Model file for the job. Use its own axes, mm. Face numbers are marked on the shaded views. A direction names the side the tool comes from. Coordinates: 2 decimals unless noted, no trailing zeros. Write each loop counter-clockwise with the first axis right and the second up, starting at its lowest first coordinate (ties: lowest second). Pieces come first, ordered by that corner, then holes.
Q1. Pin check, flat tips, straight feed: P1, Ø2.5, axis at x = -35, z = -1, coming from the -Y side; P2, Ø6, axis at x = 15.5, z = -18, coming from the -Y side; P3, Ø1, axis at x = -40.5, z = -86, coming from the -Y side; P4, Ø6, axis at x = -2.5, y = 5.5, coming from the -Z side. Stop position of each tip, or through.
Q2. Which spindle directions (+Z, -Z, +X, -X, +Y, -Y) get a long thin tool onto all of the face, cutting with end or side? Do the marked faces 5 and 6. Say none if no direction does.
Q3. Band-saw the part on C-C, the plane x = -27.5. Write the cut outline in (y, z).
Q4. Band-saw the part on D-D, the plane z = -81. Write the cut outline in (x, y).
Q5. Pull direction X, two halves, no side cores. Call the marked faces 1, 2, 3 and 4: released by +X, released by -X, zero draft, split by the parting line, or undercut.
Q6. Drill centre lines: probe 1 along X at (y, z) = (22.5, -30.5); probe 2 along Y at (x, z) = (4, -94); probe 3 along Z at (x, y) = (-5.5, 32). Where is each one in solid material? Low to high.
Q7. Band-saw the part on B-B, the plane y = 25. Write the cut outline in (x, z), plus the area to 3 significant figures.
Q8. Band-saw the part on A-A, the plane z = -7. Write the cut outline in (x, y), plus the area to 4 significant figures.
from build123d import *

# Parameters (mm, degrees)
SALIENTE_EXTRUIR1_DEPTH = 107
CROQUIS2_W              = 90
CROQUIS2_H              = 18
SALIENTE_EXTRUIR2_DEPTH = 3
CROQUIS4_W              = 90
CROQUIS4_H              = 30
SALIENTE_EXTRUIR3_DEPTH = 3
REDONDEO3_R             = 2
CROQUIS3_W              = 6
CROQUIS3_H              = 45
CORTAR_EXTRUIR1_DEPTH   = 123.776219196
REDONDEO1_R             = 5
SALIENTE_EXTRUIR4_DEPTH = 3.5
CORTAR_EXTRUIR3_START   = -3
CORTAR_EXTRUIR3_DEPTH   = 3
CORTAR_EXTRUIR4_DEPTH   = 144.589693223
SALIENTE_EXTRUIR5_DEPTH = 3
REDONDEO4_R             = 1
SALIENTE_EXTRUIR6_DEPTH = 1
CORTAR_EXTRUIR6_DEPTH   = 1


with BuildPart() as part:
    # Croquis1 → Saliente-Extruir1 (new body)
    with BuildSketch(Plane.XY):
        Polygon((-42, 0), (-45, 0), (-45, 40), (45, 40), (45, 0), (42, 0), (42, 37), (-42, 37), align=None)
    extrude(amount=-SALIENTE_EXTRUIR1_DEPTH)

    # Croquis2 → Saliente-Extruir2 (add)
    with BuildSketch(Plane(origin=(0, 0, -107), x_dir=(-1, 0, 0), z_dir=(0, 0, -1))):
        with Locations((0, 31)):
            Rectangle(CROQUIS2_W, CROQUIS2_H)
    extrude(amount=-SALIENTE_EXTRUIR2_DEPTH)

    # Croquis4 → Saliente-Extruir3 (add)
    with BuildSketch(Plane.XY):
        with Locations((0, 25)):
            Rectangle(CROQUIS4_W, CROQUIS4_H)
    extrude(amount=-SALIENTE_EXTRUIR3_DEPTH)

    # Redondeo3
    redondeo3_edges = [part.edges().sort_by_distance(p)[0] for p in [
        (0, 40, 0),
    ]]
    fillet(redondeo3_edges, radius=REDONDEO3_R)

    # Croquis3 → Cortar-Extruir1 (cut, through all)
    with BuildSketch(Plane(origin=(0, 40, 0), x_dir=(1, 0, 0), z_dir=(0, 1, 0))):
        with Locations((-9, 22.5)):
            Rectangle(CROQUIS3_W, CROQUIS3_H)
        with Locations((11, 22.5)):
            Rectangle(CROQUIS3_W, CROQUIS3_H)
        with Locations((-29, 22.5)):
            Rectangle(CROQUIS3_W, CROQUIS3_H)
        with Locations((31, 22.5)):
            Rectangle(CROQUIS3_W, CROQUIS3_H)
    extrude(amount=-CORTAR_EXTRUIR1_DEPTH, mode=Mode.SUBTRACT)

    # Redondeo1
    redondeo1_edges = [part.edges().sort_by_distance(p)[0] for p in [
        (0, 40, -107),
    ]]
    fillet(redondeo1_edges, radius=REDONDEO1_R)

    # Croquis6 → Saliente-Extruir4 (add)
    with BuildSketch(Plane(origin=(-42, 0, 0), x_dir=(0, 0, -1), z_dir=(1, 0, 0))):
        Polygon((3, 10), (0, 10), (0, 0), (107, 0), (107, 22), (104, 22), (104, 37), (3, 37), align=None)
    extrude(amount=SALIENTE_EXTRUIR4_DEPTH)

    # Croquis7 → Cortar-Extruir3 (cut)
    with BuildSketch(Plane.ZY.offset(45).offset(CORTAR_EXTRUIR3_START)):
        with BuildLine():
            Line((-2, 40), (-102, 40))
            ThreePointArc((-102, 40), (-105.535533906, 38.535533906), (-107, 35))
            Line((-107, 35), (-107, 0))
            Line((-107, 0), (0, 0))
            Line((0, 0), (0, 38))
            ThreePointArc((0, 38), (-0.585786438, 39.414213562), (-2, 40))
        make_face()
    extrude(amount=CORTAR_EXTRUIR3_DEPTH, mode=Mode.SUBTRACT)

    # Croquis8 → Cortar-Extruir4 (cut, through all)
    with BuildSketch(Plane.ZY.offset(42)):
        Polygon((-107, 0), (-94, 0), (-87, 0), (-85, 0), (-85, 4.5), (-87, 4.5), (-87, 15.5), (-94, 15.5), (-94, 20.5), (-107, 20.5), align=None)
    extrude(amount=-CORTAR_EXTRUIR4_DEPTH, mode=Mode.SUBTRACT)

    # Croquis9 → Saliente-Extruir5 (add)
    with BuildSketch(Plane(origin=(45, 0, 0), x_dir=(0, 0, -1), z_dir=(1, 0, 0))):
        with BuildLine():
            Line((10, 0), (20, 0))
            Line((20, 0), (20, -12))
            ThreePointArc((20, -12), (19.707106781, -12.707106781), (19, -13))
            Line((19, -13), (11, -13))
            ThreePointArc((11, -13), (10.292893219, -12.707106781), (10, -12))
            Line((10, -12), (10, 0))
        make_face()
    extrude(amount=-SALIENTE_EXTRUIR5_DEPTH)

    # Redondeo4
    redondeo4_edges = [part.edges().sort_by_distance(p)[0] for p in [
        (43.5, 0, -10),
        (43.5, 0, -20),
    ]]
    fillet(redondeo4_edges, radius=REDONDEO4_R)

    # Croquis11 → Saliente-Extruir6 (add)
    with BuildSketch(Plane.ZY.offset(-42)):
        with BuildLine():
            Line((-107, 20.5), (-94, 20.5))
            Line((-94, 20.5), (-94, 15.5))
            Line((-94, 15.5), (-87, 15.5))
            Line((-87, 15.5), (-87, 4.5))
            Line((-87, 4.5), (-85, 4.5))
            Line((-85, 4.5), (-85, 0))
            Line((-85, 0), (-21, 0))
            ThreePointArc((-21, 0), (-20.292893219, -0.292893219), (-20, -1))
            Line((-20, -1), (-20, -12))
            ThreePointArc((-20, -12), (-19.707106781, -12.707106781), (-19, -13))
            Line((-19, -13), (-11, -13))
            ThreePointArc((-11, -13), (-10.292893219, -12.707106781), (-10, -12))
            Line((-10, -12), (-10, -1))
            ThreePointArc((-10, -1), (-9.707106781, -0.292893219), (-9, 0))
            Line((-9, 0), (0, 0))
            Line((0, 0), (0, 10))
            Line((0, 10), (-3, 10))
            Line((-3, 10), (-3, 37))
            Line((-3, 37), (-104, 37))
            Line((-104, 37), (-104, 22))
            Line((-104, 22), (-107, 22))
            Line((-107, 22), (-107, 20.5))
        make_face()
    extrude(amount=SALIENTE_EXTRUIR6_DEPTH)

    # Croquis12 → Cortar-Extruir6 (cut)
    with BuildSketch(Plane(origin=(45, 0, 0), x_dir=(0, 0, -1), z_dir=(1, 0, 0))):
        with BuildLine():
            Line((94, 20.5), (107, 20.5))
            Line((107, 20.5), (107, 35))
            ThreePointArc((107, 35), (105.535533906, 38.535533906), (102, 40))
            Line((102, 40), (2, 40))
            ThreePointArc((2, 40), (0.585786438, 39.414213562), (0, 38))
            Line((0, 38), (0, 0))
            Line((0, 0), (9, 0))
            ThreePointArc((9, 0), (9.707106781, -0.292893219), (10, -1))
            Line((10, -1), (10, -12))
            ThreePointArc((10, -12), (10.292893219, -12.707106781), (11, -13))
            Line((11, -13), (19, -13))
            ThreePointArc((19, -13), (19.707106781, -12.707106781), (20, -12))
            Line((20, -12), (20, -1))
            ThreePointArc((20, -1), (20.292893219, -0.292893219), (21, 0))
            Line((21, 0), (85, 0))
            Line((85, 0), (85, 4.5))
            Line((85, 4.5), (87, 4.5))
            Line((87, 4.5), (87, 15.5))
            Line((87, 15.5), (94, 15.5))
            Line((94, 15.5), (94, 20.5))
        make_face()
    extrude(amount=-CORTAR_EXTRUIR6_DEPTH, mode=Mode.SUBTRACT)


solid = part.part
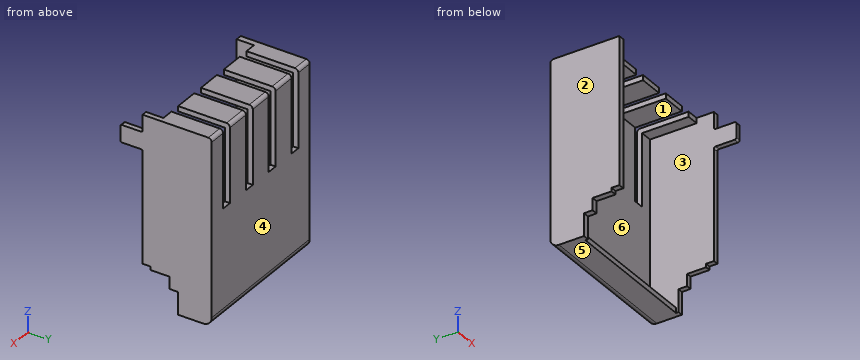
Answer sheet:
1. P1: stops at y = 10
1. P2: stops at y = 37
1. P3: stops at y = 4.5
1. P4: passes through
2. face 5: -Z, +X, -X, +Y, -Y
2. face 6: -Y
3. outline: (22, -107) - (35, -107) arc R5 ccw to (40, -102) - (40, -45) - (37, -45) - (37, -104) - (22, -104) - close
4. outline: (-42, 0) - (-38.5, 0) - (-38.5, 37) - (41, 37) - (41, 0) - (44, 0) - (44, 40) - (-42, 40) - close
5. face 1: undercut
5. face 2: released by -X
5. face 3: undercut
5. face 4: zero draft
6. probe 1: x = -42 to -38.5, 41 to 44
6. probe 2: y = 37 to 40
6. probe 3: z = -107 to -104, -3 to 0
7. outline: (-42, -107) - (44, -107) - (44, 0) - (34, 0) - (34, -3) - (41, -3) - (41, -104) - (-38.5, -104) - (-38.5, -3) - (-32, -3) - (-32, 0) - (-42, 0) - close; (-26, -3) - (-12, -3) - (-12, 0) - (-26, 0) - close; (-6, -3) - (8, -3) - (8, 0) - (-6, 0) - close; (14, -3) - (28, -3) - (28, 0) - (14, 0) - close
7. area: 1,100 mm2
8. outline: (-42, 0) - (-38.5, 0) - (-38.5, 37) - (-32, 37) - (-32, 40) - (-42, 40) - close; (-26, 37) - (-12, 37) - (-12, 40) - (-26, 40) - close; (-6, 37) - (8, 37) - (8, 40) - (-6, 40) - close; (14, 37) - (28, 37) - (28, 40) - (14, 40) - close; (34, 37) - (41, 37) - (41, 0) - (44, 0) - (44, 40) - (34, 40) - close
8. area: 426.5 mm2
